The listing builds one solid part. Answer for the finished solid, in the listing's coordinates (mm). Round coordinates to 2 decimals unless told otherwise and drop trailing zeros. Write each loop counter-clockwise with the first axis right and the second up, starting at its lowest first coordinate (ties: lowest second). Pieces come first, ordered by that corner, then holes. Notation, with made-up numbers: (-36.5, 64) - (-8.5, 64) arc R33 ccw to (-8.5, 99) - close; hole circle Ø4 at (32, 28). An arc over 180 degrees is marked (long way). Answer as CSV lines item,"result". Start each with the question number.
Item 1: A cutting plane is placed at C-C on x = 117.5. Determine the outline of the cut face in (y, z), and give its area (3 significant figures).
Item 2: Flat-ended cylindrical pins translate along their axes: pin 1 (1.7 mm diameter, centred on x = 0.5, z = 3, fed in from -Y); pin 2 (2.5 mm diameter, centred on x = 91, z = 2.5, fed in from -Y); pin 3 (2 mm diameter, centred on y = 15, z = 1.5, fed in from -X). Find the tip coordinate at first contact, or state that the pin passes through.
Item 3: A cutting plane is placed at B-B on z = 3.05. State how many separate pieces and enclosed holes the cut face has, and give its area (3 significant figures).
Item 4: Straight lines are drawn through the part: line 1 along Y through (x, z) = (0, 1.2) (3 decimals); line 2 along X through (y, z) = (-4, 0.6); line 3 along Y through (x, z) = (96.52, 1.2) (3 decimals). For each, find the intervals that lie inside material, in ascending order. Write a range as [from, to].
Item 5: A cutting plane is placed at A-A on x = 96.52. Determine the outline of the cut face in (y, z) (3 decimals), and give its area (3 significant figures).
```python
from build123d import *

# Parameters (mm, degrees)
SKETCH1_R           = 3.175
BOSS_EXTRUDE1_DEPTH = 4.7752
FILLET1_R           = 4.7752
SKETCH2_R           = 3.175
CUT_EXTRUDE2_DEPTH  = 12.6492


with BuildPart() as part:
    # Sketch1 → Boss-Extrude1 (new body)
    with BuildSketch(Plane.XY):
        with BuildLine():
            ThreePointArc((-37.394976935, 21.59), (-43.18, 0), (-37.394976935, -21.59))
            ThreePointArc((-37.394976935, -21.59), (-34.391979043, -23.934305056), (-30.603626356, -23.531630922))
            Line((-30.603626356, -23.531630922), (-12.85503117, -14.058829027))
            ThreePointArc((-12.85503117, -14.058829027), (10.51886685, -15.882567179), (17.960512242, 6.35))
            Line((17.960512242, 6.35), (152.4, 6.35))
            Line((152.4, 6.35), (152.4, 19.05))
            Line((152.4, 19.05), (0, 19.05))
            ThreePointArc((0, 19.05), (-6.89499119, 17.758423255), (-12.85503117, 14.058829027))
            Line((-12.85503117, 14.058829027), (-30.603626356, 23.531630922))
            ThreePointArc((-30.603626356, 23.531630922), (-34.391979043, 23.934305056), (-37.394976935, 21.59))
        make_face()
        with BuildLine():
            ThreePointArc((2.98992691, 5.602038653), (-1.541031238, -6.160172297), (0, 6.35))
            Line((0, 6.35), (1.588518614, 6.35))
            Line((1.588518614, 6.35), (2.98992691, 5.602038653))
        make_face(mode=Mode.SUBTRACT)
        with Locations((-38.1, 0)):
            Circle(SKETCH1_R, mode=Mode.SUBTRACT)
        with BuildLine():
            ThreePointArc((-26.946380439, -15.5575), (-31.115, 0), (-26.946380439, 15.5575))
            ThreePointArc((-26.946380439, 15.5575), (-22.609249782, 16.719630657), (-21.447119125, 12.3825))
            ThreePointArc((-21.447119125, 12.3825), (-24.765, 0), (-21.447119125, -12.3825))
            ThreePointArc((-21.447119125, -12.3825), (-22.609249782, -16.719630657), (-26.946380439, -15.5575))
        make_face(mode=Mode.SUBTRACT)
        with BuildLine():
            ThreePointArc((-18.147562336, -10.4775), (-20.955, 0), (-18.147562336, 10.4775))
            ThreePointArc((-18.147562336, 10.4775), (-13.810431679, 11.639630657), (-12.648301022, 7.3025))
            ThreePointArc((-12.648301022, 7.3025), (-14.605, 0), (-12.648301022, -7.3025))
            ThreePointArc((-12.648301022, -7.3025), (-13.810431679, -11.639630657), (-18.147562336, -10.4775))
        make_face(mode=Mode.SUBTRACT)
    extrude(amount=BOSS_EXTRUDE1_DEPTH)

    # Fillet1
    fillet1_edges = [part.edges().sort_by_distance(p)[0] for p in [
        (-12.85503117, 14.058829027, 2.3876),
        (152.4, 19.05, 2.3876),
        (152.4, 6.35, 2.3876),
        (17.960512242, 6.35, 2.3876),
        (-12.85503117, -14.058829027, 2.3876),
    ]]
    fillet(fillet1_edges, radius=FILLET1_R)

    # Sketch2 → Cut-Extrude2 (cut)
    with BuildSketch(Plane.XY.offset(4.7752)):
        with Locations((0, 12.7)):
            Circle(SKETCH2_R)
        with Locations((0, -12.7)):
            Circle(SKETCH2_R)
        with Locations((48.26, 12.7)):
            Circle(SKETCH2_R)
        with Locations((96.52, 12.7)):
            Circle(SKETCH2_R)
        with Locations((144.78, 12.7)):
            Circle(SKETCH2_R)
    extrude(amount=-CUT_EXTRUDE2_DEPTH, mode=Mode.SUBTRACT)


solid = part.part
```
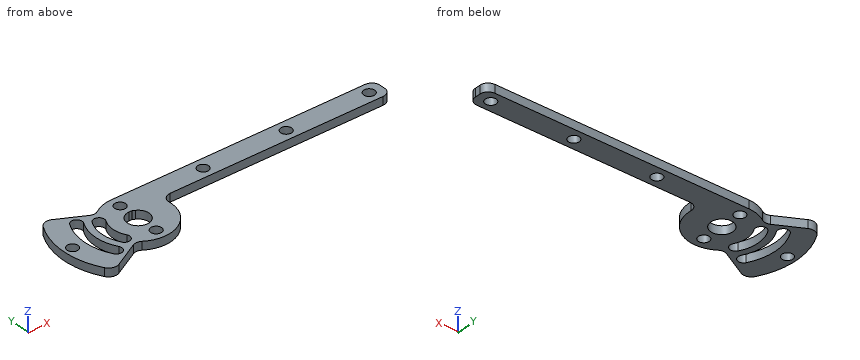
Geometry says:
1,outline,"(6.35, 0) - (19.05, 0) - (19.05, 4.78) - (6.35, 4.78) - close"
1,area,"60.6 mm^2"
2,pin 1,"stops at y = -19.05"
2,pin 2,"stops at y = 6.35"
2,pin 3,"stops at x = -40.85"
3,separate pieces,"1"
3,enclosed holes,"9"
3,area,"3,260 mm^2"
4,line 1,"y = [-19.05, -15.875], [-9.525, -6.35], [6.35, 9.525], [15.875, 19.05]"
4,line 2,"x = [-42.99, -30.86], [-24.44, -20.57], [-14.05, -4.93], [4.93, 18.63]"
4,line 3,"y = [6.35, 9.525], [15.875, 19.05]"
5,outline,"(6.35, 0) - (9.525, 0) - (9.525, 4.775) - (6.35, 4.775) - close; (15.875, 0) - (19.05, 0) - (19.05, 4.775) - (15.875, 4.775) - close"
5,area,"30.3 mm^2"
